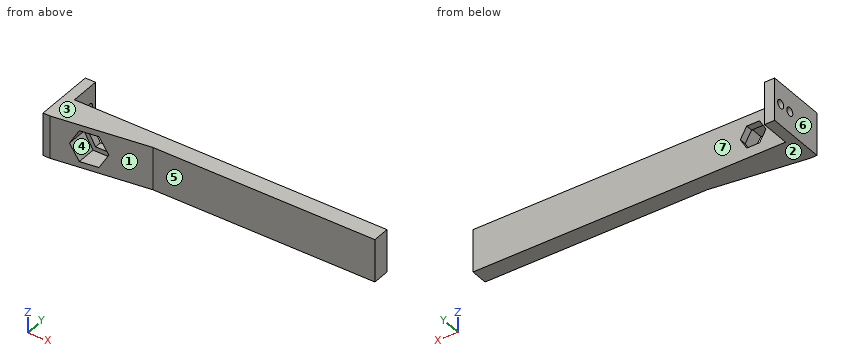
from build123d import *

# Parameters (mm, degrees)
CROQUIS3_W              = 25
CROQUIS3_H              = 35
SALIENTE_EXTRUIR2_DEPTH = 4
CROQUIS5_W              = 25
CROQUIS5_H              = 17.5
SALIENTE_EXTRUIR3_DEPTH = 2
CROQUIS7_W              = 25
CROQUIS7_H              = 10
SALIENTE_EXTRUIR5_DEPTH = 55
CROQUIS8_R              = 2.5
CORTAR_EXTRUIR1_DEPTH   = 55
SALIENTE_EXTRUIR6_DEPTH = 25
CORTAR_EXTRUIR3_DEPTH   = 4
CROQUIS11_R             = 2
CORTAR_EXTRUIR4_DEPTH   = 20
CORTAR_EXTRUIR5_DEPTH   = 45
CROQUIS13_W             = 25
CROQUIS13_H             = 10
SALIENTE_EXTRUIR7_DEPTH = 130


with BuildPart() as part:
    # Croquis3 → Saliente-Extruir2 (new body)
    with BuildSketch(Plane(origin=(0, 0, 0), x_dir=(0, 0, -1), z_dir=(1, 0, 0))):
        with Locations((4.326923077, 2.8125)):
            Rectangle(CROQUIS3_W, CROQUIS3_H)
    extrude(amount=SALIENTE_EXTRUIR2_DEPTH)

    # Croquis5 → Saliente-Extruir3 (add)
    with BuildSketch(Plane(origin=(4, 0, 0), x_dir=(0, 0, -1), z_dir=(1, 0, 0))):
        with Locations((4.326923077, 11.5625)):
            Rectangle(CROQUIS5_W, CROQUIS5_H)
    extrude(amount=SALIENTE_EXTRUIR3_DEPTH)

    # Croquis7 → Saliente-Extruir5 (add)
    with BuildSketch(Plane(origin=(4, 0, 0), x_dir=(0, 0, -1), z_dir=(1, 0, 0))):
        with Locations((4.326923077, -2.1875)):
            Rectangle(CROQUIS7_W, CROQUIS7_H)
    extrude(amount=SALIENTE_EXTRUIR5_DEPTH)

    # Croquis8 → Cortar-Extruir1 (cut)
    with BuildSketch(Plane(origin=(6, 0, 0), x_dir=(0, 0, -1), z_dir=(1, 0, 0))):
        with Locations((4.326923077, 15.3125)):
            Circle(CROQUIS8_R)
        with Locations((4.326923077, 7.8125)):
            Circle(CROQUIS8_R)
    extrude(amount=-CORTAR_EXTRUIR1_DEPTH, mode=Mode.SUBTRACT)

    # Croquis10 → Saliente-Extruir6 (add, through all)
    with BuildSketch(Plane.XY.offset(8.173076923)):
        Polygon((4, -14.6875), (59, -7.1875), (4, -7.1875), align=None)
    extrude(amount=-SALIENTE_EXTRUIR6_DEPTH)

    # Croquis9 → Cortar-Extruir3 (cut)
    with BuildSketch(Plane(origin=(0, 2.8125, 0), x_dir=(1, 0, 0), z_dir=(0, 1, 0))):
        Polygon((32.505553499, 4.326923077), (28.75277675, 10.826923077), (21.24722325, 10.826923077), (17.494446501, 4.326923077), (21.24722325, -2.173076923), (28.75277675, -2.173076923), align=None)
    extrude(amount=-CORTAR_EXTRUIR3_DEPTH, mode=Mode.SUBTRACT)

    # Croquis11 → Cortar-Extruir4 (cut)
    with BuildSketch(Plane(origin=(59, 0, 0), x_dir=(0, 0, -1), z_dir=(1, 0, 0))):
        with Locations((-1.923076923, -2.1875)):
            Circle(CROQUIS11_R)
        with Locations((10.576923077, -2.1875)):
            Circle(CROQUIS11_R)
    extrude(amount=-CORTAR_EXTRUIR4_DEPTH, mode=Mode.SUBTRACT)

    # Croquis12 → Cortar-Extruir5 (cut)
    with BuildSketch(Plane(origin=(0, -1.1875, 0), x_dir=(1, 0, 0), z_dir=(0, 1, 0))):
        Polygon((30.25388745, 13.426923077), (19.74611255, 13.426923077), (14.492225101, 4.326923077), (19.74611255, -4.773076923), (30.25388745, -4.773076923), (35.507774899, 4.326923077), align=None)
    extrude(amount=-CORTAR_EXTRUIR5_DEPTH, mode=Mode.SUBTRACT)

    # Croquis13 → Saliente-Extruir7 (add)
    with BuildSketch(Plane(origin=(59, 0, 0), x_dir=(0, 0, -1), z_dir=(1, 0, 0))):
        with Locations((4.326923077, -2.1875)):
            Rectangle(CROQUIS13_W, CROQUIS13_H)
    extrude(amount=SALIENTE_EXTRUIR7_DEPTH)


solid = part.part
Work out the finished part from the listing and answer in its coordinate system (mm). Face numbers are marked on the shaded views. A direction names the side the tool comes from. Coordinates: 2 decimals unless noted, no trailing zeros. Loops run counter-clockwise (first coordinate to the right, second up) from the corner with the lowest first, then second, coordinate; pieces in that order, holes last. Notation, with made-up numbers: M 68,77.25 L 111,77.25 A22 cw 111,109.25 Z; hole C -6,37 d6. An arc over 180 degrees is marked long. Answer in a Markdown table with one row per item. Add a question column.
1. A tool of negligible diameter and unlimited length cuts with its end or side. For the marked faces 5, 6 and 7, from which of +Z, -Z, +X, -X, +Y, -Y can it reach the whole face along a straight path? Write none if from no direction.
2. Flat-ended cylindrical pins translate along their axes: P1, Ø10, axis at x = 44, z = -12.5, coming from the +Y side; P2, Ø9, axis at y = 11, z = -3, coming from the +X side; P3, Ø5, axis at x = 58.5, z = -13, coming from the -Y side; P4, Ø4, axis at y = 15.31, z = -4.33, coming from the +X side. Find the tip coordinate at first contact, or state that the pin passes through.
3. The mould has two halves that part along Z. Classify the marked faces 1, 2, 3 and 4: pulls with the +Z half, pulls with the -Z half, needs draft (parallel to the pull), parting line crosses it, or undercut.
4. Find section A-A, the plane x = 112.5. Write down the section's boundary in (y, z).
5. Consider L1, parallel to X at y = 3, z = 5; L2, parallel to Y at x = 83, z = -2.75; L3, parallel to Y at x = 57, z = 1.5. Determine where each line is inside the solid, lowest interval first.
Reported:
| question | item | result |
|---|---|---|
| 1 | face 5 | +Z, -Z, +X, -Y |
| 1 | face 6 | +Z, -Z, -X, +Y, -Y |
| 1 | face 7 | +Z, -Z, +X, +Y |
| 2 | P1 | stops at y = 2.81 |
| 2 | P2 | stops at x = 6 |
| 2 | P3 | stops at y = -7.6 |
| 2 | P4 | passes through |
| 3 | face 1 | needs draft |
| 3 | face 2 | pulls with the -Z half |
| 3 | face 3 | pulls with the +Z half |
| 3 | face 4 | undercut |
| 4 | outline | M -7.19,-16.83 L 2.81,-16.83 L 2.81,8.17 L -7.19,8.17 Z |
| 5 | L1 | x = 0 to 6 |
| 5 | L2 | y = -7.19 to 2.81 |
| 5 | L3 | y = -7.46 to -4.14, -0.23 to 2.81 |
